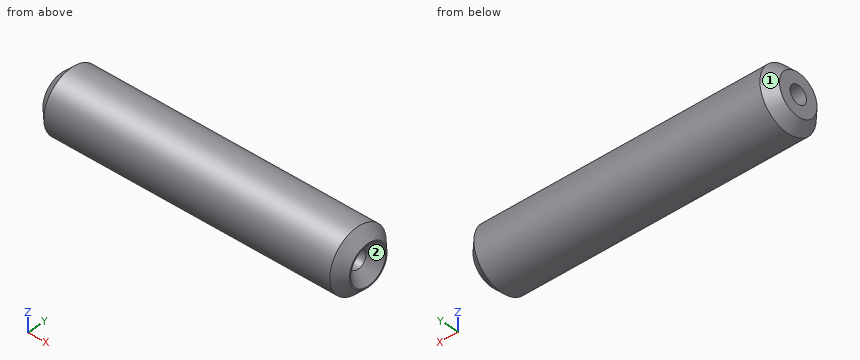
Autodesk Inventor part; units mm, degrees
ref_plane "YZ Plane" through (0, 0, 0) normal (1, 0, 0) x (0, 1, 0)
ref_plane "XZ Plane" through (0, 0, 0) normal (0, 1, 0) x (-1, 0, 0)
ref_plane "XY Plane" through (0, 0, 0) normal (0, 0, 1) x (1, 0, 0)
sketch "Szkic1" plane through (0, 0, 0) normal (1, 0, 0) x (0, 1, 0)
  circle A0 centre (0, 0) radius 3
  dimension "d0" = 6
extrude "Wyciągnięcie proste1" add sketch "Szkic1" along normal blind 30
sketch "Szkic2" plane through (30, 0, 0) normal (1, 0, 0) x (0, 0, -1)
  point P0 (0, 0)
  point P1 (0, 0)
hole "Otwór1" at (30, 0, 0) direction (-1, 0, 0) diameter 1.75 end through all
thread "Gwint1"
chamfer "Faza1" distance 1 angle 45 2 edges at (30, -3, 0) (0, -3, 0)
chamfer "Faza2" distance 1 angle 45 1 edges at (30, 0, 0.875)
properties part number "throat"
Build history of the part. All positions in model axes, mm. Face numbers are marked on the shaded views. Coordinates: 2 decimals unless noted, no trailing zeros. Write each loop counter-clockwise with the first axis right and the second up, starting at its lowest first coordinate (ties: lowest second). Pieces come first, ordered by that corner, then holes. Notation, with made-up numbers: (13, 26.25) -> (32, 26.25) arc R36 cw to (32, 63.25) -> close; hole circle Ø7 at (23, 89). An arc over 180 degrees is marked (long way). Use CSV: the item, a comma, the result in double quotes. Start each with the question number.
Q1. Cut at A-A, the plane z = 0. List the corners of the cut face in (x, y) (3 decimals), then the cut area to 4 significant figures.
Q2. Drill centre lines: probe 1 along Z at (x, y) = (12.5, 0) (3 decimals); probe 2 along Y at (x, z) = (25, -0.2); probe 3 along Z at (x, y) = (23, -0.6). Where is each one in solid material? Low to high.
Q3. Pull direction Y, two halves, no side cores. Call the marked faces 1 and 2: released by +Y, released by -Y, zero draft, split by the parting line, or undercut.
Q4. Flat gauge pins, fed straight in: pin 1 Ø3 at (y, z) = (-1, -2) entering from +X; pin 2 Ø1.1 at (y, z) = (0, 0) entering from -X; pin 3 Ø3 at (x, z) = (16, 2) entering from +Y. Where does each tip first touch, or does it go through?
Q5. Cut at C-C, the plane x = 11. List the corners of the cut face in (y, z) (3 decimals), then the cut area to 3 significant figures.
Checked values:
1,outline,"(0, -2) -> (1, -3) -> (29, -3) -> (30, -2) -> (30, -1.875) -> (29, -0.875) -> (0, -0.875) -> close; (0, 0.875) -> (29, 0.875) -> (30, 1.875) -> (30, 2) -> (29, 3) -> (1, 3) -> (0, 2) -> close"
1,area,"124.5 mm²"
2,probe 1,"z = -3 to -0.875, 0.875 to 3"
2,probe 2,"y = -2.99 to -0.85, 0.85 to 2.99"
2,probe 3,"z = -2.94 to -0.64, 0.64 to 2.94"
3,face 1,"split by the parting line"
3,face 2,"undercut"
4,pin 1,"stops at x = 30"
4,pin 2,"passes through"
4,pin 3,"stops at y = 2.96"
5,outline,"circle Ø6 at (0, 0); hole circle Ø1.75 at (0, 0)"
5,area,"25.9 mm²"
